from build123d import *

# Parameters (mm, degrees)
BOSS_EXTRU_1_DEPTH      = 5
ESQUISSE2_W             = 140
ESQUISSE2_H             = 48
ENL_V_MAT_EXTRU_1_DEPTH = 450.499721913


with BuildPart() as part:
    # Esquisse1 → Boss.-Extru.1 (new body)
    with BuildSketch(Plane.XY):
        Polygon((-200, 400), (200, 400), (200, 207.5), (205, 207.5), (205, 177.5), (200, 177.5), (200, -177.5), (205, -177.5), (205, -207.5), (200, -207.5), (200, -400), (-200, -400), (-200, -207.5), (-205, -207.5), (-205, -177.5), (-200, -177.5), (-200, 177.5), (-205, 177.5), (-205, 207.5), (-200, 207.5), align=None)
    extrude(amount=BOSS_EXTRU_1_DEPTH)

    # Esquisse2 → Enlèv. mat.-Extru.1 (cut, through all)
    with BuildSketch(Plane.XY.offset(5)):
        with Locations((0, 246)):
            Rectangle(ESQUISSE2_W, ESQUISSE2_H)
    extrude(amount=-ENL_V_MAT_EXTRU_1_DEPTH, mode=Mode.SUBTRACT)


solid = part.part
Geometry: final body of the model. Coordinates: model frame, mm. Round coordinates to 2 decimals unless told otherwise and drop trailing zeros. Order: outer loops, then holes, each group sorted by start corner. A loop starts at its lowest first (then second) coordinate and runs counter-clockwise, first axis right, second up. Notation, with made-up numbers: (-22, -16) -> (-8, -16) arc R20 cw to (-8, -6) -> close; hole circle Ø3 at (15.5, 54.5). An arc over 180 degrees is marked (long way). Put each result on its own line as item: value. Start each with the question number.
Q1. First-contact query: pin 1 (2.5 mm diameter, centred on x = 202, z = 3, fed in from -Y); pin 2 (1.5 mm diameter, centred on x = 202.5, z = 3, fed in from +Y); pin 3 (3 mm diameter, centred on x = -86.5, y = -234, fed in from -Z); pin 4 (1.5 mm diameter, centred on y = 236.5, z = 2.5, fed in from +X). Flat tips, straight axial feed; report the tip coordinate or a pass-through.
Q2. Section A-A on y = 245. Return the cut outline in (x, z).
Q3. Section B-B on x = 32. Return the cut outline in (y, z), and give its area (3 significant figures).
Q4. Section D-D on y = 41. Return the cut outline in (x, z).
Q5. Line query: probe 1 along Y at (x, z) = (-62, 3.3); probe 2 along X at (y, z) = (238, 0.4); probe 3 along X at (y, z) = (-90, 4.5). Output: solid intervals per line, ascending.
Q6. Section C-C on z = 1.7. Return the cut outline in (x, y), and give its area (3 significant figures).
Ans:
1. pin 1: stops at y = -207.5
1. pin 2: stops at y = 207.5
1. pin 3: stops at z = 0
1. pin 4: stops at x = 200
2. outline: (-200, 0) -> (-70, 0) -> (-70, 5) -> (-200, 5) -> close; (70, 0) -> (200, 0) -> (200, 5) -> (70, 5) -> close
3. outline: (-400, 0) -> (222, 0) -> (222, 5) -> (-400, 5) -> close; (270, 0) -> (400, 0) -> (400, 5) -> (270, 5) -> close
3. area: 3,760 mm2
4. outline: (-200, 0) -> (200, 0) -> (200, 5) -> (-200, 5) -> close
5. probe 1: y = -400 to 222, 270 to 400
5. probe 2: x = -200 to -70, 70 to 200
5. probe 3: x = -200 to 200
6. outline: (-205, -207.5) -> (-200, -207.5) -> (-200, -400) -> (200, -400) -> (200, -207.5) -> (205, -207.5) -> (205, -177.5) -> (200, -177.5) -> (200, 177.5) -> (205, 177.5) -> (205, 207.5) -> (200, 207.5) -> (200, 400) -> (-200, 400) -> (-200, 207.5) -> (-205, 207.5) -> (-205, 177.5) -> (-200, 177.5) -> (-200, -177.5) -> (-205, -177.5) -> close; hole (-70, 222) -> (70, 222) -> (70, 270) -> (-70, 270) -> close
6. area: 314,000 mm2
